Here's how the part is built. I have some questions about the finished solid (model axes, mm). Round coordinates to 2 decimals unless told otherwise and drop trailing zeros. Order: outer loops, then holes, each group sorted by start corner. A loop starts at its lowest first (then second) coordinate and runs counter-clockwise, first axis right, second up. Notation, with made-up numbers: (-14, 69) - (34, 69) arc R11 cw to (34, 82) - close; hole circle Ø1 at (-9.75, 14.25). An arc over 180 degrees is marked (long way). Answer as a JSON object with one key per item and string values.
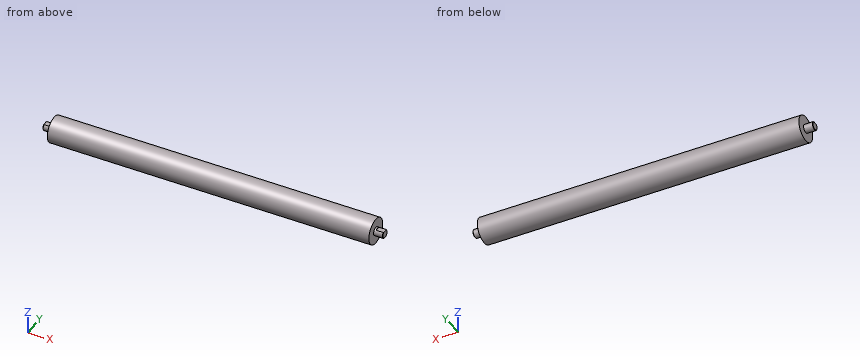
```python
from build123d import *

# Parameters (mm, degrees)
F0_R     = 27.5
F1_DEPTH = 875
F2_R     = 22.5
F3_DEPTH = 50
F5_DEPTH = 40
F6_SIZE  = 2
F8_R     = 70
F9_DEPTH = 875


with BuildPart() as f1:
    # F0 (on Right) → F1 (new body, symmetric)
    with BuildSketch(Plane.YZ):
        Circle(F0_R)
    extrude(amount=F1_DEPTH, both=True)

    # F7: F3 across plane


with BuildPart() as f3:
    # F2 (on face) → F3 (new body)
    with BuildSketch(Plane.YZ.offset(875)):
        Circle(F2_R)
    extrude(amount=F3_DEPTH)

    # F4 (on face) → F5 (cut)
    with BuildSketch(Plane.YZ.offset(925)):
        with BuildLine():
            Line((-14.142136, 17.5), (14.142136, 17.5))
            ThreePointArc((14.142136, 17.5), (0, 22.5), (-14.142136, 17.5))
        make_face()
    extrude(amount=-F5_DEPTH, mode=Mode.SUBTRACT)

    # F6
    f6_edges = [f3.edges().sort_by_distance(p)[0] for p in [
        (925, -9.696699, -20.303301),
    ]]
    chamfer(f6_edges, length=F6_SIZE)


with BuildPart() as f1_1:
    add(f1.part)
    add(f3.part.mirror(Plane.YZ))


    add(f3.part)  # F9 merges F3
    # F8 (on Right) → F9 (join, symmetric)
    with BuildSketch(Plane.YZ):
        Circle(F8_R)
    extrude(amount=F9_DEPTH, both=True)


solid = f1_1.part
```
1. Imagine slicing it at A-A (z = 0). List the corners of the cut face in (x, y) for me.
Responses:
{"outline": "(-925, -20.5) - (-923, -22.5) - (-875, -22.5) - (-875, -70) - (875, -70) - (875, -22.5) - (923, -22.5) - (925, -20.5) - (925, 20.5) - (923, 22.5) - (875, 22.5) - (875, 70) - (-875, 70) - (-875, 22.5) - (-923, 22.5) - (-925, 20.5) - close"}
2. Imagine slicing it at C-C (y = -50). List the corners of the cut face in (x, z) for me, plus the area to 3 significant figures.
Responses:
{"outline": "(-875, -48.99) - (875, -48.99) - (875, 48.99) - (-875, 48.99) - close", "area": "171,000 mm2"}
3. Imagine slicing it at B-B (x = -116). List the corners of the cut face in (y, z) for me, plus the area to 3 significant figures.
Responses:
{"outline": "circle Ø140 at (0, 0)", "area": "15,400 mm2"}
4. If I drill on L1, parallel to X at y = 18, z = -56.5; L2, parallel to Y at x = -548, z = 20; L3, parallel to Y at x = 141.5, z = -33.5, over which ranges is the centre line in solid material (lowest first)? Write a range as [from, to].
Responses:
{"L1": "[-875, 875]", "L2": "[-67.08, 67.08]", "L3": "[-61.46, 61.46]"}
5. For P1, Ø2.5, axis at y = 4, z = 20, coming from the +X side; P2, Ø1, axis at y = 41.5, z = 22.5, coming from the +X side; P3, Ø5, axis at x = 2.5, y = -52.5, coming from the -Z side; P4, Ø5.5, axis at y = 6.5, z = 20, coming from the -X side, each with a flat end and sliding along its axis, tell me the tip position at first contact or that it passes through.
Responses:
{"P1": "x = 885", "P2": "x = 875", "P3": "z = -48.99", "P4": "x = -925"}
